from build123d import *

# Parameters (mm, degrees)
SKETCH_1_R      = 5
EXTRUDE_1_DEPTH = 10


with BuildPart() as part:
    # 草图1 → 凸台-拉伸1 (new body)
    with BuildSketch(Plane(origin=(0, 0, 0), x_dir=(1, 0, 0), z_dir=(0, 1, 0))):
        Polygon((0, 18.091268752), (7.540032115, 20.716584923), (11.670850027, 18.708548438), (9.045634376, 15.667498326), (16.888151818, 14.171072765), (19.461526826, 10.366653202), (15.667498326, 9.045634376), (21.71110488, 3.828433104), (22.037503228, -0.752978388), (18.091268752, 0), (20.716584923, -7.540032115), (18.708548438, -11.670850027), (15.667498326, -9.045634376), (14.171072765, -16.888151818), (10.366653202, -19.461526826), (9.045634376, -15.667498326), (3.828433104, -21.71110488), (-0.752978388, -22.037503228), (0, -18.091268752), (-7.540032115, -20.716584923), (-11.670850027, -18.708548438), (-9.045634376, -15.667498326), (-16.888151818, -14.171072765), (-19.461526826, -10.366653202), (-15.667498326, -9.045634376), (-21.71110488, -3.828433104), (-22.037503228, 0.752978388), (-18.091268752, 0), (-20.716584923, 7.540032115), (-18.708548438, 11.670850027), (-15.667498326, 9.045634376), (-14.171072765, 16.888151818), (-10.366653202, 19.461526826), (-9.045634376, 15.667498326), (-3.828433104, 21.71110488), (0.752978388, 22.037503228), align=None)
        with Locations(Location((0, 0, 0), (0, 0, 270))):
            Circle(SKETCH_1_R, mode=Mode.SUBTRACT)
    extrude(amount=EXTRUDE_1_DEPTH)


solid = part.part
Model file for the job. Use its own axes, mm. A direction names the side the tool comes from. Round coordinates to 2 decimals unless told otherwise and drop trailing zeros. Order: outer loops, then holes, each group sorted by start corner. A loop starts at its lowest first (then second) coordinate and runs counter-clockwise, first axis right, second up. Notation, with made-up numbers: M -18.5,-20.75 L 18.5,-20.75 A24 ccw 18.5,4.25 Z; hole C 56.25,54.5 d7. An arc over 180 degrees is marked long. Write each question's results on one line, items separated by ' | '. Start each with the question number.
(1) Two-plate mould, pull along X, no slides. Class faces 1 (the face through (-18.65, 4.93, 6.47)), 2 (the face through (-3.717, 4.93, 19.386)), 3 (the face through (17.591, 4.93, -9.715)), 4 (the face through (-4.88, 4.93, -1.08)): pulls with the +X half, pulls with the -X half, needs draft (parallel to the pull), parting line crosses it, or undercut.
(2) Saw through at B-B, the plane x = 13. Give the cut face in (y, z).
(3) Which spindle directions (+Z, -Z, +X, -X, +Y, -Y) get a long thin tool onto all of the face, cutting with end or side? Do faces 5 (the face through (-17.591, 4.93, 9.715)), 6 (the face through (0.3, 0, -5.2)), 7 (the face through (-9.715, 4.93, -17.591)), 8 (the face through (12.91, 4.93, -14.93)). Say none if no direction does.
(4) Probe probe 1 along X at (y, z) = (8.75, 3); probe 2 along Z at (x, y) = (17.5, 4.25); probe 3 along Z at (x, y) = (-16.5, 5.5). List the from-to ranges inside material, lowest first. Write a range as from..to.
(5) Drop flat-ended pins along their axis: pin 1 (1.5 mm diameter, centred on x = -5, y = 8, fed in from -Z); pin 2 (1 mm diameter, centred on y = 9, z = 9, fed in from +X); pin 3 (5 mm diameter, centred on x = -17, y = 3.5, fed in from +Z); pin 4 (5 mm diameter, centred on x = -1.5, z = -1, fed in from -Y). Give the stop position or say it passes through.
(6) Saw through at A-A, the plane x = -3. Give the cut face in (y, z).
(7) Saw through at C-C, the plane x = -12.5. Give the cut face in (y, z), then the cut area to 3 significant figures.
Established:
1) face 1: pulls with the -X half | face 2: undercut | face 3: pulls with the +X half | face 4: undercut
2) outline: M 0,-14.91 L 10,-14.91 L 10,17.68 L 0,17.68 Z
3) face 5: -X, +Y, -Y | face 6: +Z, -Z, +X, -X, -Y | face 7: -Z, +Y, -Y | face 8: +X, +Y, -Y
4) probe 1: x = -21.77..-4, 4..19.14 | probe 2: z = -13.27..-9.68, -7.46..10.63 | probe 3: z = -9.76..8.33, 9.34..14.25
5) pin 1: stops at z = -21.22 | pin 2: stops at x = 20.25 | pin 3: stops at z = 14.63 | pin 4: passes through
6) outline: M 0,-21.77 L 10,-21.77 L 10,-4 L 0,-4 Z; M 0,4 L 10,4 L 10,19.14 L 0,19.14 Z
7) outline: M 0,-18.02 L 10,-18.02 L 10,15.01 L 0,15.01 Z | area: 330 mm^2
